CAD build for the part. Positions are in the model's coordinates, mm. Coordinates: 2 decimals unless noted, no trailing zeros. Loops run counter-clockwise (first coordinate to the right, second up) from the corner with the lowest first, then second, coordinate; pieces in that order, holes last. Notation, with made-up numbers: M 22,-10 L 60,-10 A22 cw 60,2 Z; hole C -22.75,-1.5 d7. An arc over 180 degrees is marked long. Answer as a JSON object with one key per item and string values. Group by question number.
Autodesk Inventor part; units mm, degrees
ref_plane "YZ Plane" through (0, 0, 0) normal (1, 0, 0) x (0, 1, 0)
ref_plane "XZ Plane" through (0, 0, 0) normal (0, 1, 0) x (-1, 0, 0)
ref_plane "XY Plane" through (0, 0, 0) normal (0, 0, 1) x (1, 0, 0)
sketch "Sketch_1" plane through (0, 0, 0) normal (0, 0, 1) x (1, 0, 0)
  line L0 (-114.3, 37.084) -> (-114.3, 0)
  line L1 (-114.3, 0) -> (0, 0)
  line L2 (0, 0) -> (0, 114.3)
  line L3 (0, 114.3) -> (-37.084, 114.3)
  line L4 (-37.084, 114.3) -> (-37.084, 40.259)
  arc A0 (-40.259, 37.084) -> (-37.084, 40.259) centre (-40.259, 40.259) ccw
  line L5 (-40.259, 37.084) -> (-114.3, 37.084)
  circle A1 centre (-19.05, 19.05) radius 4.1656
  circle A2 centre (-19.05, 95.25) radius 4.1656
  circle A3 centre (-19.05, 57.15) radius 4.1656
  circle A4 centre (-57.15, 19.05) radius 4.1656
  circle A5 centre (-95.25, 19.05) radius 4.1656
extrude "Extrusion1" add sketch "Sketch_1" along normal blind 6.35
properties part number "4481"
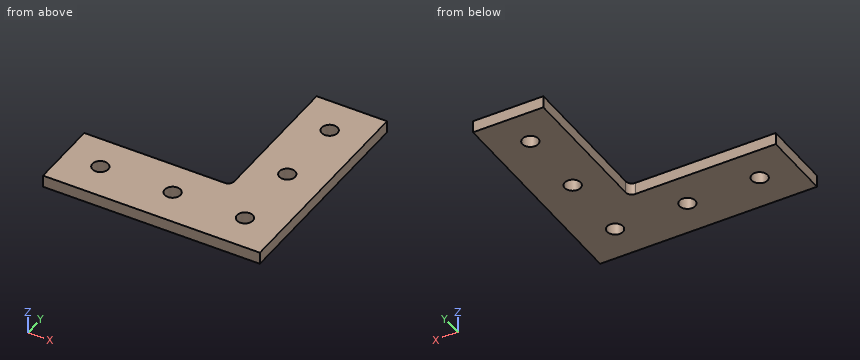
Item 1: Drill centre lines: L1, parallel to Y at x = -19.05, z = 2.75; L2, parallel to X at y = 19.5, z = 2; L3, parallel to Y at x = -95.25, z = 4.75. Where is each one in solid material? Low to high. Write a range as from..to.
Item 2: Slice it at D-D, the plane y = 19.05. Write the cut outline in (x, z), then the cut area to 3 significant figures.
Item 3: Slice it at B-B, the plane y = 95.25. Write the cut outline in (x, z), then the cut area to 3 significant figures.
Item 4: Slice it at A-A, the plane x = -57.15. Write the cut outline in (y, z), then the cut area to 3 significant figures.
Item 5: Slice it at C-C, the plane x = -19.05. Write the cut outline in (y, z).
Item 6: Pin check, flat tips, straight feed: pin 1 (1 mm diameter, centred on y = 68.5, z = 5.5, fed in from -X); pin 2 (3 mm diameter, centred on x = -91, z = 4, fed in from +Y); pin 3 (11 mm diameter, centred on x = -19.05, y = 57.15, fed in from -Z). Stop position of each tip, or through.
Computed:
{
 "1": {"L1": "0..14.88, 23.22..52.98, 61.32..91.08, 99.42..114.3", "L2": "-114.3..-99.39, -91.11..-61.29, -53.01..-23.19, -14.91..0", "L3": "0..14.88, 23.22..37.08"},
 "2": {"outline": "M -114.3,0 L -99.42,0 L -99.42,6.35 L -114.3,6.35 Z; M -91.08,0 L -61.32,0 L -61.32,6.35 L -91.08,6.35 Z; M -52.98,0 L -23.22,0 L -23.22,6.35 L -52.98,6.35 Z; M -14.88,0 L 0,0 L 0,6.35 L -14.88,6.35 Z", "area": "567 mm2"},
 "3": {"outline": "M -37.08,0 L -23.22,0 L -23.22,6.35 L -37.08,6.35 Z; M -14.88,0 L 0,0 L 0,6.35 L -14.88,6.35 Z", "area": "183 mm2"},
 "4": {"outline": "M 0,0 L 14.88,0 L 14.88,6.35 L 0,6.35 Z; M 23.22,0 L 37.08,0 L 37.08,6.35 L 23.22,6.35 Z", "area": "183 mm2"},
 "5": {"outline": "M 0,0 L 14.88,0 L 14.88,6.35 L 0,6.35 Z; M 23.22,0 L 52.98,0 L 52.98,6.35 L 23.22,6.35 Z; M 61.32,0 L 91.08,0 L 91.08,6.35 L 61.32,6.35 Z; M 99.42,0 L 114.3,0 L 114.3,6.35 L 99.42,6.35 Z"},
 "6": {"pin 1": "x = -37.08", "pin 2": "y = 37.08", "pin 3": "z = 0"}
}
